Source: CAD feature listing. Evaluate the final solid. Frame: model axes, mm. Face numbers are marked on the shaded views. A direction names the side the tool comes from. Give positions to 0.01 mm unless a question says otherwise; leave off trailing zeros. Order: outer loops, then holes, each group sorted by start corner. A loop starts at its lowest first (then second) coordinate and runs counter-clockwise, first axis right, second up. Notation, with made-up numbers: M -14,70.5 L 23,70.5 A37 cw 23,106.5 Z; hole C 32.25,25 d5. An arc over 180 degrees is marked long. Return JSON: item names as keys, results as strings.
from build123d import *

# Parameters (mm, degrees)
F0_W     = 5.37864
F0_H     = 3.654586
F1_DEPTH = 50
F3_D     = 3
F4_SIZE  = 2


with BuildPart() as f1:
    # F0 (on Front) → F1 (new body)
    with BuildSketch(Plane.XZ):
        Polygon((-2.704546, -5), (-2.704546, 0), (2.704546, 0), (2.704546, -5), (4.704546, -4.963173), (4.704546, 1.118637), (4.704546, 2), (4.361257, 2), (2.68932, 2), (-2.68932, 2), (-4.704546, 2), (-4.704546, 1.118637), (-4.704546, -4.963173), align=None)
        with Locations((0, 3.827293)):
            Rectangle(F0_W, F0_H)
    extrude(amount=-F1_DEPTH)

    # F3 (through all)
    with Locations(Plane.XZ):
        with Locations((0, 3.068567)):
            Hole(F3_D / 2)

    # F4
    f4_edges = [f1.edges().sort_by_distance(p)[0] for p in [
        (2.68932, 25, 2),
        (-2.68932, 25, 2),
    ]]
    chamfer(f4_edges, length=F4_SIZE)


solid = f1.part
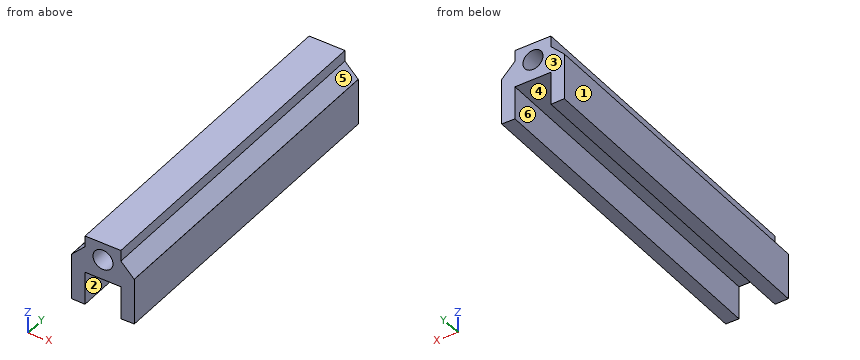
1. First-contact query: pin 1 (1.6 mm diameter, centred on x = 0, y = 33, fed in from -Z); pin 2 (0.8 mm diameter, centred on y = 14.5, z = 4.5, fed in from +X); pin 3 (1.3 mm diameter, centred on y = 16.5, z = 5, fed in from -X). Flat tips, straight axial feed; report the tip coordinate or a pass-through.
Evaluation:
{"pin 1": "stops at z = 0", "pin 2": "stops at x = 2.69", "pin 3": "stops at x = -2.69"}
2. Section query C-C (z = 3.5). Return loops of the section in (x, y).
Evaluation:
{"outline": "M -3.19,0 L -1.44,0 L -1.44,50 L -3.19,50 Z; M 1.44,0 L 3.19,0 L 3.19,50 L 1.44,50 Z"}
3. Set-up query: the marked faces 1 and 2. Return all of +Z, -Z, +X, -X, +Y, -Y with unobstructed straight access to the full face (end or side cutting, diameter ignored); none if empty.
Evaluation:
{"face 1": "+Z, -Z, -X, +Y, -Y", "face 2": "-Z, +Y, -Y"}
4. Section query D-D (x = -3.25). Return loops of the section in (y, z), then the cut area to 3 significant figures.
Evaluation:
{"outline": "M 0,-4.99 L 50,-4.99 L 50,3.44 L 0,3.44 Z", "area": "421 mm^2"}
5. Section query A-A (x = 0). Return loops of the section in (y, z).
Evaluation:
{"outline": "M 0,0 L 50,0 L 50,1.57 L 0,1.57 Z; M 0,4.57 L 50,4.57 L 50,5.65 L 0,5.65 Z"}
6. Draft query along X for the marked faces 3, 4, 5 and 6. Return one class per face: pulls with the +X half, pulls with the -X half, needs draft (parallel to the pull), parting line crosses it, or undercut.
Evaluation:
{"face 3": "needs draft", "face 4": "undercut", "face 5": "pulls with the +X half", "face 6": "undercut"}
7. Ray query, probe 1 along X at (y, z) = (2, -3.25); probe 2 along Z at (x, y) = (0, 25); probe 3 along X at (y, z) = (36, 2). Return the intervals inside material, ascending.
Evaluation:
{"probe 1": "x = -4.7 to -2.7, 2.7 to 4.7", "probe 2": "z = 0 to 1.57, 4.57 to 5.65", "probe 3": "x = -4.69 to -1.05, 1.05 to 4.69"}
